```python
from build123d import *

# Parameters (mm, degrees)
F0_R     = 19.05
F1_DEPTH = 63.5
F2_R     = 5.5626
F3_DEPTH = 61.9262
F4_DEPTH = 4.7752
F5_DEPTH = 61.9262


with BuildPart() as f1:
    # F0 (on Front) → F1 (new body)
    with BuildSketch(Plane.XZ):
        with BuildLine():
            Line((38.1, 28.575), (0, 28.575))
            ThreePointArc((0, 28.575), (-19.345366451, -21.0306305629), (28.4756083945, 2.38125))
            ThreePointArc((28.4756083945, 2.38125), (30.9572676717, 9.6234554837), (37.9674778593, 12.7))
            Line((37.9674778593, 12.7), (96.8502, 12.7))
            Line((96.8502, 12.7), (96.8502, 33.3502))
            Line((96.8502, 33.3502), (38.1, 33.3502))
            Line((38.1, 33.3502), (38.1, 28.575))
        make_face()
        Circle(F0_R, mode=Mode.SUBTRACT)
    extrude(amount=F1_DEPTH)

    # F2 (on face) → F3 (cut, through all)
    with BuildSketch(Plane.XY.offset(33.3502)):
        with Locations((50.8, -50.8)):
            Circle(F2_R)
        with Locations((50.8, -12.7)):
            Circle(F2_R)
        with Locations((84.1502, -31.75)):
            Circle(F2_R)
    extrude(amount=-F3_DEPTH, mode=Mode.SUBTRACT)

    # F2 (on face) → F4 (cut)
    with BuildSketch(Plane.XY.offset(33.3502)):
        with BuildLine():
            ThreePointArc((38.1, -12.7), (41.8197438789, -3.7197438789), (50.8, 0))
            Line((50.8, 0), (38.1, 0))
            Line((38.1, 0), (38.1, -12.7))
        make_face()
        with BuildLine():
            Line((38.1, -63.5), (50.8, -63.5))
            ThreePointArc((50.8, -63.5), (41.8197438789, -59.7802561211), (38.1, -50.8))
            Line((38.1, -50.8), (38.1, -63.5))
        make_face()
    extrude(amount=-F4_DEPTH, mode=Mode.SUBTRACT)

    # F2 (on face) → F5 (cut, through all)
    with BuildSketch(Plane.XY.offset(33.3502)):
        with BuildLine():
            ThreePointArc((96.8502, -31.75), (95.1340352623, -38.1253715915), (90.4493554441, -42.7777214642))
            Line((90.4493554441, -42.7777214642), (57.0991554441, -61.8277214642))
            ThreePointArc((57.0991554441, -61.8277214642), (54.0586759125, -63.0748128824), (50.8, -63.5))
            Line((50.8, -63.5), (96.8502, -63.5))
            Line((96.8502, -63.5), (96.8502, -31.75))
        make_face()
        with BuildLine():
            ThreePointArc((90.4493554441, -20.7222785358), (95.1340352623, -25.3746284085), (96.8502, -31.75))
            Line((96.8502, -31.75), (96.8502, 0))
            Line((96.8502, 0), (50.8, 0))
            ThreePointArc((50.8, 0), (54.0586759125, -0.4251871176), (57.0991554441, -1.6722785358))
            Line((57.0991554441, -1.6722785358), (90.4493554441, -20.7222785358))
        make_face()
    extrude(amount=-F5_DEPTH, mode=Mode.SUBTRACT)


solid = f1.part
```
The listing builds one solid part. Answer for the finished solid, in the listing's coordinates (mm). A direction names the side the tool comes from. Coordinates: 2 decimals unless noted, no trailing zeros. Loops run counter-clockwise (first coordinate to the right, second up) from the corner with the lowest first, then second, coordinate; pieces in that order, holes last. Notation, with made-up numbers: (-14.5, 18) -> (41.5, 18) arc R20 cw to (41.5, 33) -> close; hole circle Ø3 at (89, 81). An arc over 180 degrees is marked (long way). Use one line per item in the form item = value. Start each with the question number.
Item 1: Consider L1, parallel to Z at x = 0, y = -18.5 (3 decimals); L2, parallel to Y at x = 50, z = 18; L3, parallel to Z at x = 80, y = -40.5. Determine where each line is inside the solid, lowest interval first. Write a range as [from, to].
Item 2: The mould has two halves that part along Y. Classify faces 1 (the face through (20, -31, 28.575)), 2 (the face through (53.79, -8.01, 23.17)), 3 (the face through (19, 0, 7)): released by +Y, released by -Y, zero draft, split by the parting line, or undercut.
Item 3: The part is cut by section D-D on y = -24. Determine the outline of the cut face in (x, z) (3 decimals), then the cut area to 3 significant figures.
Item 4: A tool of negligible diameter and unlimited length cuts with its end or side. For faces 4 (the face through (61, -31, 33.35)), 5 (the face through (38.1, -31, 31)), 6 (the face through (60, -31, 12.7)), from which of +Z, -Z, +X, -X, +Y, -Y can it reach the whole face along a straight path? Write none if from no direction.
Item 5: Flat-ended cylindrical pins translate along their axes: pin 1 Ø6 at (y, z) = (-44.5, -7.5) entering from +X; pin 2 Ø1 at (y, z) = (-50.5, -6.5) entering from -X; pin 3 Ø2 at (y, z) = (-47.5, -8.5) entering from -X. Find the tip coordinate at first contact, or state that the pin passes through.
Item 6: The part is cut by section A-A on z = 0. Determine the outline of the cut face in (x, y) (3 decimals), then the cut area to 3 significant figures.
Item 7: The part is cut by section B-B on y = -15.5. Count the separate pieces of the cut face and the enclosed holes in it, then the cut area to 3 significant figures.
Item 8: The part is cut by section C-C on x = 14.5. Determine the outline of the cut face in (y, z) (3 decimals), then the cut area to 3 significant figures.
Answer key:
q1.L1 = [-28.575, -19.05], [19.05, 28.575]
q1.L2 = [-63.5, -56.3], [-45.3, -18.2], [-7.2, 0]
q1.L3 = [12.7, 33.35]
q2.face_1 = zero draft
q2.face_2 = undercut
q2.face_3 = released by +Y
q3.outline = (0, 28.575) arc R28.575 ccw (long way) to (28.476, 2.381) arc R9.525 cw to (37.967, 12.7) -> (94.211, 12.7) -> (94.211, 33.35) -> (38.1, 33.35) -> (38.1, 28.575) -> close; hole circle Ø38.1 at (0, 0)
q3.area = 2,930 mm2
q4.face_4 = +Z, +X, -X, +Y, -Y
q4.face_5 = +Z, -X, +Y, -Y
q4.face_6 = -Z, +X, +Y, -Y
q5.pin_1 = 28.22
q5.pin_2 = -27.94
q5.pin_3 = -27.57
q6.outline = (-28.575, -63.5) -> (-19.05, -63.5) -> (-19.05, 0) -> (-28.575, 0) -> close; (19.05, -63.5) -> (28.575, -63.5) -> (28.575, 0) -> (19.05, 0) -> close
q6.area = 1,210 mm2
q7.separate_pieces = 2
q7.enclosed_holes = 1
q7.area = 2,460 mm2
q8.outline = (-63.5, -24.623) -> (0, -24.623) -> (0, -12.355) -> (-63.5, -12.355) -> close; (-63.5, 12.355) -> (0, 12.355) -> (0, 28.575) -> (-63.5, 28.575) -> close
q8.area = 1,810 mm2
